Input: part model. Units: mm. Frame: model coordinates. A direction names the side the tool comes from. Give positions to 0.01 mm unless a question says otherwise; leave off trailing zeros. Order: outer loops, then holes, each group sorted by start corner. A loop starts at its lowest first (then second) coordinate and runs counter-clockwise, first axis right, second up. Notation, with made-up numbers: (63.25, 12.5) - (107.25, 12.5) arc R3 cw to (107.25, 17.5) - close; hole circle Ø11 at (43.5, 71). An arc over 180 degrees is marked (long way). Use a Markdown table: item, result.
from build123d import *

# Parameters (mm, degrees)
BOX004_W     = 63
BOX004_H     = 37
BOX004_DEPTH = 5
BOX003_W     = 10
BOX003_H     = 8
BOX003_DEPTH = 5


with BuildPart() as cube004:
    # Box004 → Box004 (new body)
    with BuildSketch(Plane.XY):
        with Locations((31.5, 18.5)):
            Rectangle(BOX004_W, BOX004_H)
    extrude(amount=BOX004_DEPTH)


with BuildPart() as battery_model001:
    # Box003 → Box003 (new body)
    with BuildSketch(Plane(origin=(63, 16, 0), x_dir=(1, 0, 0), z_dir=(0, 0, 1))):
        with Locations((5, 4)):
            Rectangle(BOX003_W, BOX003_H)
    extrude(amount=BOX003_DEPTH)

    # Fusion001: union Cube004
    add(cube004.part)


with BuildPart() as battery_model001_1:
    # Fusion001 placement: moved
    add(battery_model001.part.moved(Location((3, 3, 3))))


solid = battery_model001_1.part
1. Pin query (flat end, axial travel): pin 1 (2.5 mm diameter, centred on y = 13.5, z = 5.5, fed in from +X); pin 2 (2.5 mm diameter, centred on x = 71.5, z = 6.5, fed in from -Y). Return the tip coordinate at first contact, or that it passes through.
Response:
| item | result |
|---|---|
| pin 1 | stops at x = 66 |
| pin 2 | stops at y = 19 |
2. Material intervals for line 1 along X through (y, z) = (5, 7.35); line 2 along Y through (x, z) = (73, 3.95), sorted ascending.
Response:
| item | result |
|---|---|
| line 1 | x = 3 to 66 |
| line 2 | y = 19 to 27 |
3. Section query B-B (y = 29). Return loops of the section in (x, z).
Response:
| item | result |
|---|---|
| outline | (3, 3) - (66, 3) - (66, 8) - (3, 8) - close |
4. Section query A-A (z = 4.55). Return loops of the section in (x, y).
Response:
| item | result |
|---|---|
| outline | (3, 3) - (66, 3) - (66, 19) - (76, 19) - (76, 27) - (66, 27) - (66, 40) - (3, 40) - close |
5. Set-up query: faces 1 (the face through (71, 19, 5)), 2 (the face through (71, 27, 5)), 3 (the face through (76, 23, 5)). Return all of +Z, -Z, +X, -X, +Y, -Y with unobstructed straight access to the full face (end or side cutting, diameter ignored); none if empty.
Response:
| item | result |
|---|---|
| face 1 | +Z, -Z, +X, -Y |
| face 2 | +Z, -Z, +X, +Y |
| face 3 | +Z, -Z, +X, +Y, -Y |
